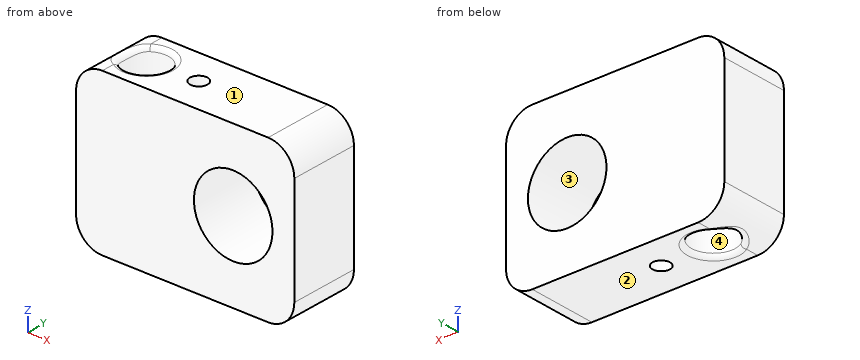
```python
from build123d import *

# Parameters (mm, degrees)
SKETCH1_W                  = 25
SKETCH1_H                  = 18.26
BOSS_EXTRUDE1_DEPTH        = 4
M10X1_0_TAPPED_HOLE1_D     = 9
M10X1_0_TAPPED_HOLE1_DEPTH = 25
M10X1_0_TAPPED_HOLE1_TIP   = 2.703872786
CUT_EXTRUDE1_DEPTH         = 16.987710906
CUT_EXTRUDE1_DEPTH_BACK    = 16.987710906
SKETCH4_R                  = 2.5
SKETCH4_R_2                = 1
FILLET1_R                  = 3
FILLET2_R                  = 0.5


with BuildPart() as part:
    # Sketch1 → Boss-Extrude1 (new, symmetric)
    with BuildSketch(Plane(origin=(0, 0, 0), x_dir=(1, 0, 0), z_dir=(0, 1, 0))):
        Rectangle(SKETCH1_W, SKETCH1_H)
    extrude(amount=BOSS_EXTRUDE1_DEPTH, both=True)

    # M10x1.0 Tapped Hole1
    with Locations(Plane(origin=(0, 4, 0), x_dir=(-1, 0, 0), z_dir=(0, 1, 0))):
        with Locations((-5.5, 0)):
            Hole(M10X1_0_TAPPED_HOLE1_D / 2, depth=M10X1_0_TAPPED_HOLE1_DEPTH)
            with Locations((0, 0, -(M10X1_0_TAPPED_HOLE1_DEPTH + M10X1_0_TAPPED_HOLE1_TIP / 2))):  # 118° drill point
                Cone(0, M10X1_0_TAPPED_HOLE1_D / 2, M10X1_0_TAPPED_HOLE1_TIP, mode=Mode.SUBTRACT)

    # Sketch4 → Cut-Extrude1 (cut, two sides: drawn at the far end of the back side and taken through both)
    with BuildSketch(Plane.XY.offset(-CUT_EXTRUDE1_DEPTH_BACK)):
        with Locations((-7.84, 0)):
            Circle(SKETCH4_R)
        with Locations((-1.86, 0)):
            Circle(SKETCH4_R_2)
    extrude(amount=CUT_EXTRUDE1_DEPTH + CUT_EXTRUDE1_DEPTH_BACK, mode=Mode.SUBTRACT)

    # Fillet1
    # the kernel refuses this fillet: 3 mm, written as the material it takes off along each edge
    with BuildSketch(Plane(origin=(-12.5, -11.5, -9.13), x_dir=(1, 0, 0), z_dir=(0, 1, 0)), Plane(origin=(12.5, 11.5, -9.13), x_dir=(-1, 0, 0), z_dir=(0, -1, 0))) as fillet1_piece_1:
        with BuildLine():
            CenterArc((FILLET1_R, -FILLET1_R), FILLET1_R, 90, 90)
            Line((0, -FILLET1_R), (0, 0))
            Line((0, 0), (FILLET1_R, 0))
        make_face()
    extrude(amount=23, mode=Mode.SUBTRACT)
    with BuildSketch(Plane(origin=(12.5, 11.5, 9.13), x_dir=(-1, 0, 0), z_dir=(0, -1, 0)), Plane(origin=(-12.5, -11.5, 9.13), x_dir=(1, 0, 0), z_dir=(0, 1, 0))) as fillet1_piece_2:
        with BuildLine():
            CenterArc((FILLET1_R, FILLET1_R), FILLET1_R, 180, 90)
            Line((0, FILLET1_R), (0, 0))
            Line((0, 0), (FILLET1_R, 0))
        make_face()
    extrude(amount=23, mode=Mode.SUBTRACT)

    # Fillet2
    fillet2_edges = [part.edges().sort_by_distance(p)[0] for p in [
        (-6.815304923, 2.28035085, -9.13),
        (-6.815304923, -2.28035085, 9.13),
        (-10.34, 0, 9.01),
        (-10.34, 0, -9.01),
    ]]
    fillet(fillet2_edges, radius=FILLET2_R)


solid = part.part
```
Input: part model. Units: mm. Frame: model coordinates. Face numbers are marked on the shaded views. Round coordinates to 2 decimals unless told otherwise and drop trailing zeros. Loops run counter-clockwise (first coordinate to the right, second up) from the corner with the lowest first, then second, coordinate; pieces in that order, holes last. Notation, with made-up numbers: (-5.75, 64) - (18.25, 64) arc R6 cw to (18.25, 68) - close; hole circle Ø5 at (-21, -15). An arc over 180 degrees is marked (long way). One line per item, written item: value. Start each with the question number.
(1) Draft query along Z for the marked faces 1, 2, 3 and 4. Return one class per face: +Z half, -Z half, draft (parallel to the pull), parting line (faces both ways), or undercut.
(2) Section A-A, the plane z = 0. Return loops of the section in (x, y).
(3) Contact query for a flat-ended pin moving along its axis: P1, Ø6, axis at x = 8.5, z = -0.5, coming from the +Y side. Output: stop coordinate, or through.
(4) Section C-C, the plane z = -2. Return loops of the section in (x, y).
(5) Section D-D, the plane x = -1.86. Return loops of the section in (y, z), plus the area to 3 significant figures.
(6) Ray query, line 1 (X direction, y = 0, z = -0.25); line 2 (Y direction, x = -7.75, z = -0.25); line 3 (X direction, y = 0, z = -4.75). Return the intervals inside material, ascending. Write a range as [from, to].
(7) Section B-B, the plane x = 5.5. Return loops of the section in (y, z), plus the area to 3 significant figures.
Results below:
1. face 1: +Z half
1. face 2: -Z half
1. face 3: undercut
1. face 4: draft
2. outline: (-12.5, -4) - (1, -4) - (1, 4) - (-12.5, 4) - close; (10, -4) - (12.5, -4) - (12.5, 4) - (10, 4) - close; hole circle Ø5 at (-7.84, 0); hole circle Ø2 at (-1.86, 0)
3. P1: y = 4
4. outline: (-12.5, -4) - (1.47, -4) - (1.47, 4) - (-12.5, 4) - close; (9.53, -4) - (12.5, -4) - (12.5, 4) - (9.53, 4) - close; hole circle Ø5 at (-7.84, 0); hole circle Ø2 at (-1.86, 0)
5. outline: (-4, -9.13) - (-1, -9.13) - (-1, 9.13) - (-4, 9.13) - close; (1, -9.13) - (4, -9.13) - (4, 9.13) - (1, 9.13) - close
5. area: 110 mm^2
6. line 1: [-12.5, -10.34], [-5.34, -2.86], [-0.86, 1.01], [9.99, 12.5]
6. line 2: [-4, -2.5], [2.5, 4]
6. line 3: [-12.5, -10.34], [-5.34, -2.86], [-0.86, 12.5]
7. outline: (-4, -9.13) - (4, -9.13) - (4, -4.5) - (-4, -4.5) - close; (-4, 4.5) - (4, 4.5) - (4, 9.13) - (-4, 9.13) - close
7. area: 74.1 mm^2
